Part print with two shaded views. Sizes in mm from the minimum x, y, z corner. A direction names the side the tool comes from. Round coordinates to 2 decimals unless told otherwise and drop trailing zeros. Order: outer loops, then holes, each group sorted by start corner. A loop starts at its lowest first (then second) coordinate and runs counter-clockwise, first axis right, second up. Notation, with made-up numbers: M 21.5,63.5 L 29.5,63.5 A14 cw 29.5,74.5 Z; hole C -4.5,48.5 d8. An arc over 180 degrees is marked long. Return JSON: item names as keys, results as strings. Group by question number.
Item 1: Pin check, flat tip, straight feed: pin 1 Ø1 at (x, y) = (81.5, 55) entering from +Z. Stop position of the tip, or through.
Item 2: Slice it at D-D on x = 107.5. Write the cut outline in (y, z), then the cut area to 3 significant figures.
Item 3: Which spindle directions (+Z, -Z, +X, -X, +Y, -Y) get a long thin tool onto all of the face, cutting with end or side? Do the marked faces 1 and 2. Say none if no direction does.
Item 4: Probe line 1 along Z through (x, y) = (3, 50.75); line 2 along X through (y, z) = (55, 34); line 3 along Y through (x, z) = (94, 9.5). List the from-to ranges inside material, lowest first.
Item 5: Slice it at C-C on z = 12. Write the cut outline in (x, y), then the cut area to 3 significant figures.
Item 6: Pull direction X, two halves, no side cores. Call the marked faces 3, 4 and 5: pulls with the +X half, pulls with the -X half, needs draft (parallel to the pull), parting line crosses it, or undercut.
Item 7: Slice it at A-A on z = 47.5. Write the cut outline in (x, y).
Item 8: Slice it at B-B on y = 50.75. Write the cut outline in (x, z), then the cut area to 3 significant figures.
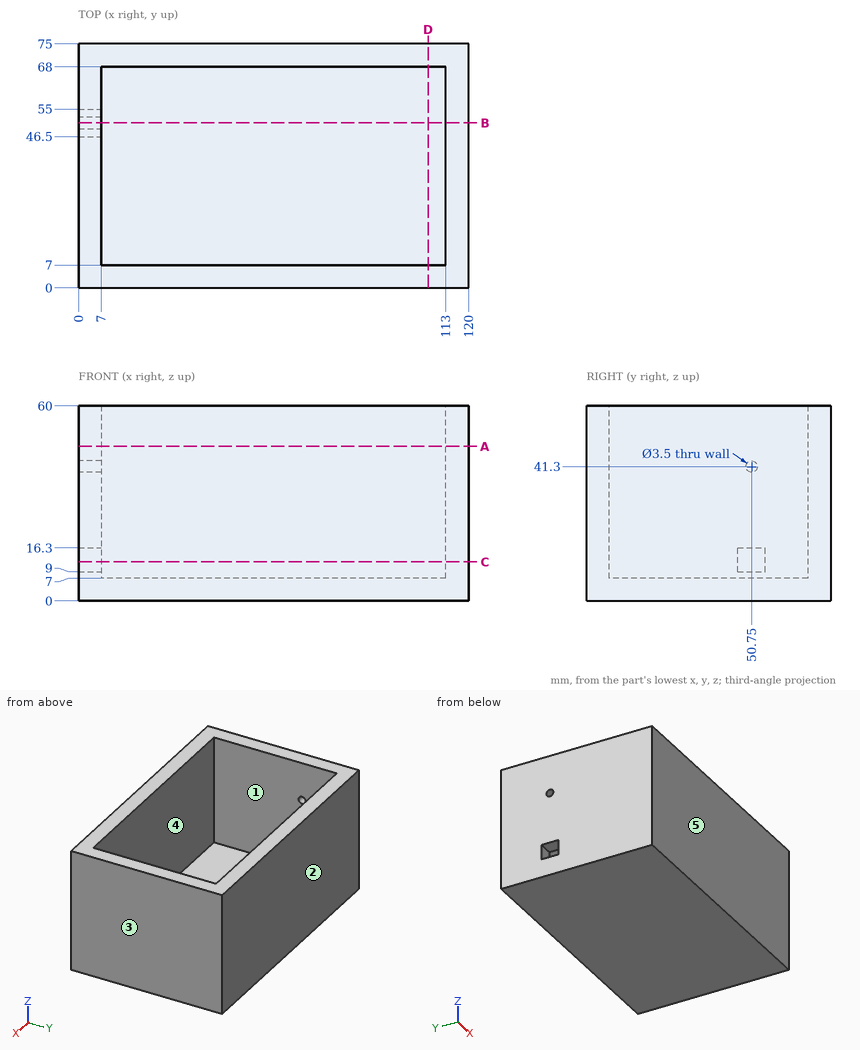
Output values:
{
 "1": {"pin 1": "z = 7"},
 "2": {"outline": "M 0,0 L 75,0 L 75,60 L 68,60 L 68,7 L 7,7 L 7,60 L 0,60 Z", "area": "1,270 mm²"},
 "3": {"face 1": "+Z", "face 2": "+Z, -Z, +X, -X, +Y"},
 "4": {"line 1": "0 to 9, 16.3 to 39.55, 43.05 to 60", "line 2": "0 to 7, 113 to 120", "line 3": "0 to 7, 68 to 75"},
 "5": {"outline": "M 0,0 L 120,0 L 120,75 L 0,75 L 0,55 L 7,55 L 7,68 L 113,68 L 113,7 L 7,7 L 7,46.5 L 0,46.5 Z", "area": "2,470 mm²"},
 "6": {"face 3": "pulls with the +X half", "face 4": "undercut", "face 5": "needs draft"},
 "7": {"outline": "M 0,0 L 120,0 L 120,75 L 0,75 Z; hole M 7,7 L 113,7 L 113,68 L 7,68 Z"},
 "8": {"outline": "M 0,0 L 120,0 L 120,60 L 113,60 L 113,7 L 7,7 L 7,9 L 0,9 Z; M 0,16.3 L 7,16.3 L 7,39.55 L 0,39.55 Z; M 0,43.05 L 7,43.05 L 7,60 L 0,60 Z", "area": "1,510 mm²"}
}
